Check sheet for the modelled part. Datum: model origin and axes. Units: mm. A direction names the side the tool comes from. Coordinates: 2 decimals unless noted, no trailing zeros. Write each loop counter-clockwise with the first axis right and the second up, starting at its lowest first coordinate (ties: lowest second). Pieces come first, ordered by that corner, then holes. Notation, with made-up numbers: (78.5, -11) - (122.5, -11) arc R32 ccw to (122.5, 18) - close; hole circle Ø2 at (38, 19). An arc over 180 degrees is marked (long way). Write each question's results on one line, items separated by ' | '.
from build123d import *

# Parameters (mm, degrees)
CUT_EXTRUDE_START   = -12
CUT_EXTRUDE_1_DEPTH = 12
CUT_EXTRUDE_2_DEPTH = 12
CHAMFER_1_SIZE      = 5
CHAMFER_2_SIZE      = 2


with BuildPart() as part:
    # Эскиз1 → Повернуть1 (revolve)
    with BuildSketch(Plane(origin=(0, 0, 0), x_dir=(-1, 0, 0), z_dir=(0, 0, -1)), mode=Mode.PRIVATE) as revolve_1_sk:
        Polygon((-13.5, -224), (0, -224), (0, 0), (-18, 0), (-18, -17.5), (-13.5, -22), align=None)
    revolve(revolve_1_sk.sketch.rotate(Axis((0, -224, 0), (0, 1, 0)), 270), axis=Axis((0, -224, 0), (0, 1, 0)))

    # Эскиз2 → Вырез-Вытянуть1 (cut)
    with BuildSketch(Plane(origin=(0, 0, 0), x_dir=(-1, 0, 0), z_dir=(0, 1, 0)).offset(CUT_EXTRUDE_START)):
        with BuildLine():
            Line((-12.449899598, 13), (12.449899598, 13))
            ThreePointArc((12.449899598, 13), (0, 18), (-12.449899598, 13))
        make_face()
    extrude(amount=CUT_EXTRUDE_1_DEPTH, mode=Mode.SUBTRACT)

    # Эскиз3 → Вырез-Вытянуть2 (cut)
    with BuildSketch(Plane(origin=(0, 0, 0), x_dir=(-1, 0, 0), z_dir=(0, 1, 0)).offset(CUT_EXTRUDE_START)):
        with BuildLine():
            Line((12.449899598, -13), (-12.449899598, -13))
            ThreePointArc((-12.449899598, -13), (0, -18), (12.449899598, -13))
        make_face()
    extrude(amount=CUT_EXTRUDE_2_DEPTH, mode=Mode.SUBTRACT)

    # Фаска1
    chamfer_1_edges = [part.edges().sort_by_distance(p)[0] for p in [
        (-18, 0, 0),
        (18, 0, 0),
    ]]
    chamfer(chamfer_1_edges, length=CHAMFER_1_SIZE - 0.0001)  # a hair under: the kernel refuses the full size

    # Фаска2
    chamfer_2_edges = [part.edges().sort_by_distance(p)[0] for p in [
        (0, -224, -13.5),
    ]]
    chamfer(chamfer_2_edges, length=CHAMFER_2_SIZE)


solid = part.part
1. Sectioned sample at A-A (z = 0). Record the cut outline in (x, y), then the cut area to 3 significant figures.
Values follow:
outline: (-18, -17.5) - (-13.5, -22) - (-13.5, -222) - (-11.5, -224) - (11.5, -224) - (13.5, -222) - (13.5, -22) - (18, -17.5) - (18, -5) - (13, 0) - (-13, 0) - (-18, -5) - close | area: 6,200 mm^2
2. Material ranges on L1, parallel to Z at x = -7, y = -45; L2, parallel to Z at x = -0.5, y = -9, recorded low to high. Write a range as [from, to].
Values follow:
L1: z = [-11.54, 11.54] | L2: z = [-13, 13]
3. Sectioned sample at B-B (y = -148.5). Record the cut outline in (x, z).
Values follow:
outline: circle Ø27 at (0, 0)
4. Access from +Z, -Z, +X, -X, +Y, -Y to the whole of each face (thin tool, end or side, straight path). Record for faces 1 (the flat face through (0, -7, -13)), 2 (the cylindrical face through (-13.18, -123.4, -2.93)), 3 (the flat face through (0, -12, 15)).
Values follow:
face 1: -Z, +X, -X, +Y | face 2: -Y | face 3: +Z, +X, -X, +Y
5. Go/stop test with flat-tipped pins: pin 1 (4 mm diameter, centred on x = -14, y = -28.5, fed in from -Z); pin 2 (5 mm diameter, centred on y = -140, z = 12, fed in from -X); pin 3 (12 mm diameter, centred on x = -14.5, y = -176.5, fed in from +Z). Record where each tip stops, or that it passes through.
Values follow:
pin 1: stops at z = -6.18 | pin 2: stops at x = -9.59 | pin 3: stops at z = 10.49
